from build123d import *

# Parameters (mm, degrees)
F0_R      = 2.5
F1_DEPTH  = 8
F3_DEPTH  = 6
F4_R      = 4.6
F4_R_2    = 2.5
F5_DEPTH  = 1.5
F6_R      = 14
F7_DEPTH  = 19.2
F9_DEPTH  = 16.5
F11_DEPTH = 20


with BuildPart() as f1:
    # F0 (on Top) → F1 (new body)
    with BuildSketch(Plane.XY):
        Circle(F0_R)
    extrude(amount=F1_DEPTH)

    # F2 (on face) → F3 (cut)
    with BuildSketch(Plane(origin=(0, 0, 0), x_dir=(1, 0, 0), z_dir=(0, 0, -1))):
        with BuildLine():
            Line((-1.475, -2.018508), (-1.475, 2.018508))
            ThreePointArc((-1.475, 2.018508), (-2.5, 0), (-1.475, -2.018508))
        make_face()
        with BuildLine():
            ThreePointArc((1.475, -2.018508), (2.5, 0), (1.475, 2.018508))
            Line((1.475, 2.018508), (1.475, -2.018508))
        make_face()
    extrude(amount=-F3_DEPTH, mode=Mode.SUBTRACT)

    # F4 (on face) → F5 (join)
    with BuildSketch(Plane.XY.offset(8)):
        Circle(F4_R)
        Circle(F4_R_2, mode=Mode.SUBTRACT)
        Circle(F4_R_2)
    extrude(amount=F5_DEPTH)

    # F6 (on face) → F7 (join)
    with BuildSketch(Plane.XY.offset(9.5)):
        with Locations((0, 7.6)):
            Circle(F6_R)
    extrude(amount=F7_DEPTH)

    # F8 (on face) → F9 (join)
    with BuildSketch(Plane(origin=(0, 0, 9.5), x_dir=(1, 0, 0), z_dir=(0, 0, -1))):
        with BuildLine():
            ThreePointArc((7.25, -19.57654), (0, -21.6), (-7.25, -19.57654))
            Line((-7.25, -19.57654), (-7.25, -24.07654))
            Line((-7.25, -24.07654), (7.25, -24.07654))
            Line((7.25, -24.07654), (7.25, -19.57654))
        make_face()
    extrude(amount=-F9_DEPTH)


with BuildPart() as f11:
    # F10 (on face) → F11 (new body)
    with BuildSketch(Plane(origin=(0, 0, 6), x_dir=(1, 0, 0), z_dir=(0, 0, -1))):
        with BuildLine():
            Line((-1.25, -4.426906), (-1.25, -42.481614))
            ThreePointArc((-1.25, -42.481614), (0, -42.5), (1.25, -42.481614))
            Line((1.25, -42.481614), (1.25, -4.426906))
            ThreePointArc((1.25, -4.426906), (3.252642, -3.252741), (4.426868, -1.250135))
            Line((4.426868, -1.250135), (42.48161, -1.250135))
            ThreePointArc((42.48161, -1.250135), (42.5, -0.000135), (42.481618, 1.249865))
            Line((42.481618, 1.249865), (4.426945, 1.249865))
            ThreePointArc((4.426945, 1.249865), (3.252741, 3.252642), (1.25, 4.426906))
            Line((1.25, 4.426906), (1.25, 42.481614))
            ThreePointArc((1.25, 42.481614), (0, 42.5), (-1.25, 42.481614))
            Line((-1.25, 42.481614), (-1.25, 4.426906))
            ThreePointArc((-1.25, 4.426906), (-3.252741, 3.252642), (-4.426945, 1.249865))
            Line((-4.426945, 1.249865), (-42.481618, 1.249865))
            ThreePointArc((-42.481618, 1.249865), (-42.5, -0.000135), (-42.48161, -1.250135))
            Line((-42.48161, -1.250135), (-4.426868, -1.250135))
            ThreePointArc((-4.426868, -1.250135), (-3.252642, -3.252741), (-1.25, -4.426906))
        make_face()
    extrude(amount=F11_DEPTH)

    # F12: cut F1
    add(f1.part, mode=Mode.SUBTRACT)


solid = f11.part
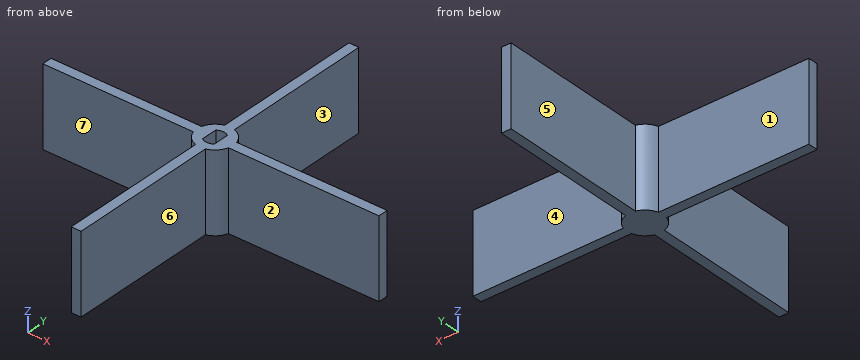
Geometry check sheet. Reference: the model listing, model coordinates, mm. Face numbers are marked on the shaded views. A direction names the side the tool comes from. Coordinates: 2 decimals unless noted, no trailing zeros. Write each loop counter-clockwise with the first axis right and the second up, starting at its lowest first coordinate (ties: lowest second). Pieces come first, ordered by that corner, then holes. Notation, with made-up numbers: (4.25, 34) -> (48.25, 34) arc R23 ccw to (48.25, 46) -> close; hole circle Ø9 at (59.5, -1.75). An arc over 180 degrees is marked (long way). One line per question, with ' | ' between items.
1. Cross-section at C-C on z = -6.75. Record the cut outline in (x, y), and give its area (3 significant figures).
Answers:
outline: (-42.48, -1.25) -> (-4.43, -1.25) arc R4.6 ccw to (-1.25, -4.43) -> (-1.25, -42.48) arc R42.5 ccw to (1.25, -42.48) -> (1.25, -4.43) arc R4.6 ccw to (4.43, -1.25) -> (42.48, -1.25) arc R42.5 ccw to (42.48, 1.25) -> (4.43, 1.25) arc R4.6 ccw to (1.25, 4.43) -> (1.25, 42.48) arc R42.5 ccw to (-1.25, 42.48) -> (-1.25, 4.43) arc R4.6 ccw to (-4.43, 1.25) -> (-42.48, 1.25) arc R42.5 ccw to start | area: 446 mm²
2. Draft check along Y on the marked faces 1, 2 and 3. Enter one of: +Y half, -Y half, draft (parallel to the pull), parting line (faces both ways), or undercut.
Answers:
face 1: +Y half | face 2: -Y half | face 3: draft
3. Depth check by flat-ended pin: pin 1 Ø1 at (y, z) = (15, 0.5) entering from -X; pin 2 Ø10 at (y, z) = (23, -7.5) entering from +X; pin 3 Ø1.2 at (y, z) = (0, 3.5) entering from -X. Enter the tip coordinate at first touch or a pass-through.
Answers:
pin 1: stops at x = -1.25 | pin 2: stops at x = 1.25 | pin 3: stops at x = -42.5
4. Set-up check for the marked faces 4, 5, 6 and 7: record each of +Z, -Z, +X, -X, +Y, -Y from which the full face is reachable in a straight line by a thin tool's end or side.
Answers:
face 4: +Z, -Z, +X, +Y | face 5: +Z, -Z, -X, +Y | face 6: +Z, -Z, +X, -Y | face 7: +Z, -Z, -X, -Y
5. Thickness scan on probe 1 along Y at (x, z) = (28, 3.75). Record the ranges inside material, lowest first. Write a range as from..to.
Answers:
probe 1: y = -1.25..1.25
6. Cross-section at D-D on y = 27. Record the cut outline in (x, z), and give its area (3 significant figures).
Answers:
outline: (-1.25, -14) -> (1.25, -14) -> (1.25, 6) -> (-1.25, 6) -> close | area: 50.0 mm²
7. Cross-section at B-B on x = 0. Record the cut outline in (y, z), and give its area (3 significant figures).
Answers:
outline: (-42.5, -14) -> (42.5, -14) -> (42.5, 6) -> (2.5, 6) -> (2.5, 0) -> (-2.5, 0) -> (-2.5, 6) -> (-42.5, 6) -> close | area: 1,670 mm²
